Verification items for this drawing (mm, ordinates from the low corner). Round coordinates to 2 decimals unless told otherwise and drop trailing zeros. Loops run counter-clockwise (first coordinate to the right, second up) from the corner with the lowest first, then second, coordinate; pieces in that order, holes last. Notation, with made-up numbers: (-23.5, 23.25) -> (-2.5, 23.25) arc R32 ccw to (-2.5, 59.25) -> close; hole circle Ø6 at (23, 69.25). An arc over 180 degrees is marked (long way). One line per item, written item: value. Start each with the question number.
1. Release check for a two-part mould opening along X. For the marked faces 1, 2 and 3 record: +X half, -X half, draft (parallel to the pull), parting line (faces both ways), or undercut.
2. Material ranges on L1, parallel to X at y = 458, z = 208; L2, parallel to Y at x = 210.5, z = 188.5; L3, parallel to Z at x = 446.5, y = 241, recorded low to high.
3. Cross-section at A-A on y = 364. Record the cut outline in (x, z), then the cut area to 3 significant figures.
4. Cross-section at B-B on x = 94. Record the cut outline in (y, z).
5. Cross-section at C-C on z = 173. Record the cut outline in (x, y).
6. Cross-section at D-D on x = 288. Record the cut outline in (y, z), then the cut area to 3 significant figures.
7. Go/stop test with flat-tipped pins: pin 1 (12.5 mm diameter, centred on x = 429.5, z = 176, fed in from +Y); pin 2 (1 mm diameter, centred on y = 390, z = 38.5, fed in from -X); pin 3 (15 mm diameter, centred on y = 390, z = 195, fed in from +X). Record where each tip stops, or that it passes through.
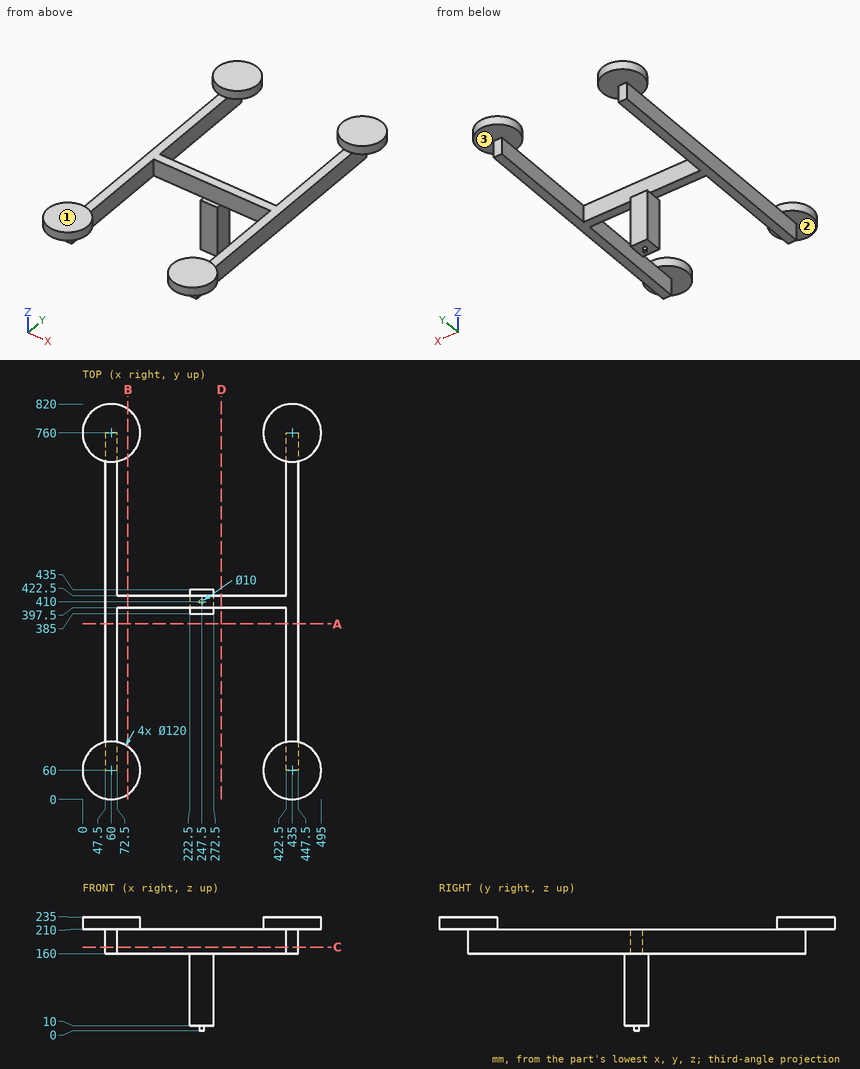
Taken from the geometry:
1. face 1: draft
1. face 2: undercut
1. face 3: undercut
2. L1: x = 47.5 to 72.5, 422.5 to 447.5
2. L2: y = 397.5 to 422.5
2. L3: z = 160 to 210
3. outline: (47.5, 160) -> (72.5, 160) -> (72.5, 210) -> (47.5, 210) -> close; (422.5, 160) -> (447.5, 160) -> (447.5, 210) -> (422.5, 210) -> close
3. area: 2,500 mm2
4. outline: (10.56, 210) -> (109.44, 210) -> (109.44, 235) -> (10.56, 235) -> close; (397.5, 160) -> (422.5, 160) -> (422.5, 210) -> (397.5, 210) -> close; (710.56, 210) -> (809.44, 210) -> (809.44, 235) -> (710.56, 235) -> close
5. outline: (47.5, 60) -> (72.5, 60) -> (72.5, 397.5) -> (422.5, 397.5) -> (422.5, 60) -> (447.5, 60) -> (447.5, 760) -> (422.5, 760) -> (422.5, 422.5) -> (72.5, 422.5) -> (72.5, 760) -> (47.5, 760) -> close
6. outline: (397.5, 160) -> (422.5, 160) -> (422.5, 210) -> (397.5, 210) -> close
6. area: 1,250 mm2
7. pin 1: stops at y = 760
7. pin 2: stops at x = 222.5
7. pin 3: stops at x = 447.5
